```python
from build123d import *

# Parameters (mm, degrees)
SKETCH_1_W          = 150
SKETCH_1_H          = 150
EXTRUDE_1_DEPTH     = 33
SKETCH_2_W          = 138
SKETCH_2_H          = 138
CUT_EXTRUDE_1_DEPTH = 12
SKETCH_3_W          = 130
SKETCH_3_H          = 130
CUT_EXTRUDE_2_DEPTH = 6
SKETCH_4_W          = 110
SKETCH_4_H          = 110
CUT_EXTRUDE_3_DEPTH = 109.124927746


with BuildPart() as part:
    # Эскиз1 → Бобышка-Вытянуть1 (new body)
    with BuildSketch(Plane(origin=(0, 0, 0), x_dir=(1, 0, 0), z_dir=(0, 1, 0))):
        Rectangle(SKETCH_1_W, SKETCH_1_H)
    extrude(amount=EXTRUDE_1_DEPTH)

    # Эскиз2 → Вырез-Вытянуть1 (cut)
    with BuildSketch(Plane(origin=(0, 33, 0), x_dir=(1, 0, 0), z_dir=(0, 1, 0))):
        Rectangle(SKETCH_2_W, SKETCH_2_H)
    extrude(amount=-CUT_EXTRUDE_1_DEPTH, mode=Mode.SUBTRACT)

    # Эскиз3 → Вырез-Вытянуть2 (cut)
    with BuildSketch(Plane(origin=(0, 0, 0), x_dir=(-1, 0, 0), z_dir=(0, -1, 0))):
        Rectangle(SKETCH_3_W, SKETCH_3_H)
    extrude(amount=-CUT_EXTRUDE_2_DEPTH, mode=Mode.SUBTRACT)

    # Эскиз4 → Вырез-Вытянуть3 (cut, through all)
    with BuildSketch(Plane(origin=(0, 21, 0), x_dir=(1, 0, 0), z_dir=(0, 1, 0))):
        Rectangle(SKETCH_4_W, SKETCH_4_H)
    extrude(amount=-CUT_EXTRUDE_3_DEPTH, mode=Mode.SUBTRACT)


solid = part.part
```
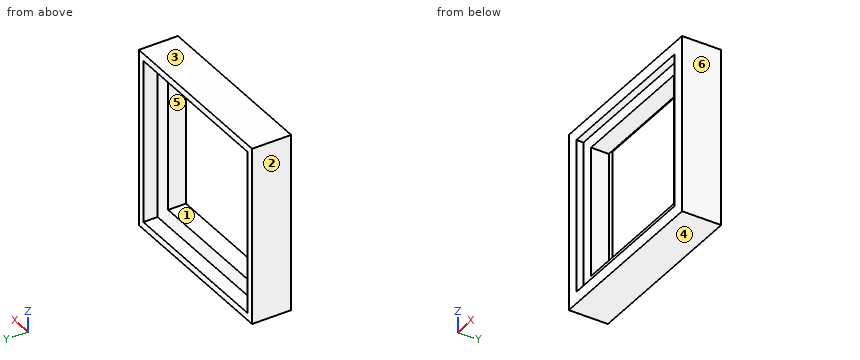
Can you work these out from the model? Positions are in its coordinate system, mm. Face numbers are marked on the shaded views. A direction names the side the tool comes from. Give positions to 0.01 mm unless a question says otherwise; leave off trailing zeros. Order: outer loops, then holes, each group sorted by start corner. A loop starts at its lowest first (then second) coordinate and runs counter-clockwise, first axis right, second up. Notation, with made-up numbers: M 6.25,30 L 29.25,30 A28 cw 29.25,63 Z; hole C 39.5,29 d10. An arc over 180 degrees is marked long. One line per item, written item: value.
1) For P1, Ø8, axis at x = 51.5, z = 21.5, coming from the -Y side; P2, Ø6, axis at x = 59.5, z = 56, coming from the +Y side; P3, Ø2, axis at x = 53, z = -18.5, coming from the +Y side, each with a flat end and sliding along its axis, tell me the tip position at first contact or that it passes through.
Answer sheet:
P1: stops at y = 6
P2: stops at y = 21
P3: passes through
2) On a 3-axis mill with a long thin cutter (end or side, diameter ignored), from which of +Z, -Z, +X, -X, +Y, -Y can I reach the whole of each face in a straight line? I mean the marked faces 5 and 6. Say none if no direction works.
Answer sheet:
face 5: +Y, -Y
face 6: +Z, -Z, +X, +Y, -Y
3) I want a section at C-C, the plane y = 17. List the corners of the cut face in (x, z) for me, plus the area to 3 significant figures.
Answer sheet:
outline: M -75,-75 L 75,-75 L 75,75 L -75,75 Z; hole M -55,-55 L 55,-55 L 55,55 L -55,55 Z
area: 10,400 mm^2
4) I want a section at A-A, the plane z = 30. List the corners of the cut face in (x, y) for me.
Answer sheet:
outline: M -75,0 L -65,0 L -65,6 L -55,6 L -55,21 L -69,21 L -69,33 L -75,33 Z; M 55,6 L 65,6 L 65,0 L 75,0 L 75,33 L 69,33 L 69,21 L 55,21 Z
5) We'd pull the mould along Z, two halves only. Please class the marked faces 1, 2, 3 and 4: released by +Z, released by -Z, zero draft, split by the parting line, or undercut.
Answer sheet:
face 1: undercut
face 2: zero draft
face 3: released by +Z
face 4: released by -Z
6) I want a section at D-D, the plane x = 57. List the corners of the cut face in (y, z) for me.
Answer sheet:
outline: M 0,-75 L 33,-75 L 33,-69 L 21,-69 L 21,69 L 33,69 L 33,75 L 0,75 L 0,65 L 6,65 L 6,-65 L 0,-65 Z
7) I want a section at B-B, the plane x = -20. List the corners of the cut face in (y, z) for me, plus the area to 3 significant figures.
Answer sheet:
outline: M 0,-75 L 33,-75 L 33,-69 L 21,-69 L 21,-55 L 6,-55 L 6,-65 L 0,-65 Z; M 0,65 L 6,65 L 6,55 L 21,55 L 21,69 L 33,69 L 33,75 L 0,75 Z
area: 864 mm^2
8) Please list where these lines run through material, in increasing order: line 1 along X through (y, z) = (8.5, -41.5); line 2 along Z through (x, y) = (-1, 29).
Answer sheet:
line 1: x = -75 to -55, 55 to 75
line 2: z = -75 to -69, 69 to 75
